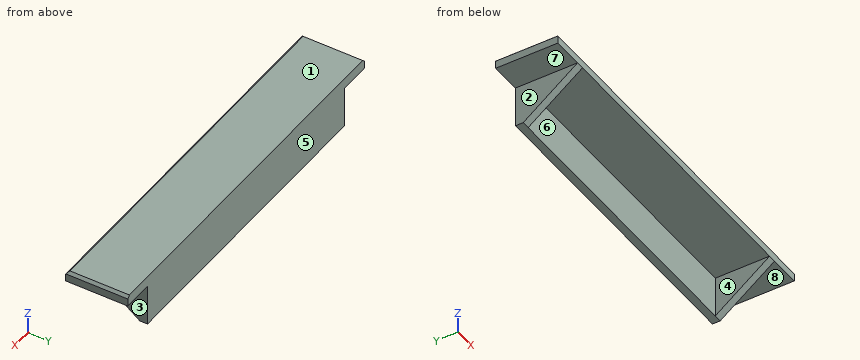
```python
from build123d import *

# Parameters (mm, degrees)
F0_W     = 914.4
F0_H     = 25.4
F1_DEPTH = 152.4
F2_SIZE  = 6.35
F3_W     = 19.05
F3_H     = 152.4
F4_DEPTH = 101.6
F6_DEPTH = 838.201
F7_W     = 19.05
F7_H     = 101.6
F8_DEPTH = 723.9


with BuildPart() as f1:
    # F0 (on Front) → F1 (new body)
    with BuildSketch(Plane.XZ):
        Rectangle(F0_W, F0_H)
    extrude(amount=F1_DEPTH)

    # F2
    f2_edges = [f1.edges().sort_by_distance(p)[0] for p in [
        (-457.2, -76.2, 12.7),
        (0, -152.4, 12.7),
        (457.2, -76.2, 12.7),
    ]]
    chamfer(f2_edges, length=F2_SIZE)

    # F3 (on face) → F4 (join)
    with BuildSketch(Plane(origin=(0, 0, -12.7), x_dir=(1, 0, 0), z_dir=(0, 0, -1))):
        with Locations((-371.475, 76.2)):
            Rectangle(F3_W, F3_H)
        with Locations((371.475, 76.2)):
            Rectangle(F3_W, F3_H)
    extrude(amount=F4_DEPTH)

    # F5 (on face) → F6 (cut, through all)
    with BuildSketch(Plane.YZ.offset(381)):
        Polygon((-19.05, -114.3), (-152.4, -12.7), (-152.4, -114.3), align=None)
    extrude(amount=-F6_DEPTH, mode=Mode.SUBTRACT)

    # F7 (on face) → F8 (join, through all)
    with BuildSketch(Plane.YZ.offset(-361.95)):
        with Locations((-9.525, -63.5)):
            Rectangle(F7_W, F7_H)
    extrude(amount=F8_DEPTH)


solid = f1.part
```
Read the model definition and answer for the solid it produces. Units are mm, in the model's axes. Face numbers are marked on the shaded views. A direction names the side the tool comes from. Give positions to 0.01 mm unless a question says otherwise; leave off trailing zeros. Loops run counter-clockwise (first coordinate to the right, second up) from the corner with the lowest first, then second, coordinate; pieces in that order, holes last.
Item 1: The part is cut by section A-A (z = -37.5). Write down the section's boundary in (x, y).
Item 2: Each of these flat-tipped pins is pushed along its axis until it touches: pin 1 Ø8 at (y, z) = (-15.5, -53.5) entering from -X; pin 2 Ø1.5 at (x, z) = (-191.5, -49.5) entering from -Y; pin 3 Ø3 at (x, y) = (305, -114.5) entering from -Z. Where does it stop, or does it pass through?
Item 3: The part is cut by section B-B (x = -189). Write down the section's boundary in (y, z), and give its area (3 significant figures).
Item 4: The part is cut by section D-D (x = 394). Write down the section's boundary in (y, z), and give its area (3 significant figures).
Item 5: Find the intervals of material crossed by line 1 along X through (y, z) = (-20, -34.5); line 2 along Z through (x, y) = (96.5, -59); line 3 along Y through (x, z) = (17, -22.5), in increasing order.
Item 6: The mould has two halves that part along X. Classify the marked faces 1, 2, 3 and 4: released by +X, released by -X, zero draft, split by the parting line, or undercut.
Item 7: For the marked faces 5, 6, 7 and 8, determine the directions among +Z, -Z, +X, -X, +Y, -Y from which every point of the face is accessible in a straight line to the end or side of a thin tool.
Item 8: The part is cut by section C-C (y = -114). Write down the section's boundary in (x, z).
Taken from the geometry:
1. outline: (-381, -119.85) - (-361.95, -119.85) - (-361.95, -19.05) - (361.95, -19.05) - (361.95, -119.85) - (381, -119.85) - (381, 0) - (-381, 0) - close
2. pin 1: stops at x = -381
2. pin 2: stops at y = -19.05
2. pin 3: stops at z = -12.7
3. outline: (-152.4, -12.7) - (-19.05, -12.7) - (-19.05, -114.3) - (0, -114.3) - (0, 12.7) - (-146.05, 12.7) - (-152.4, 6.35) - close
3. area: 5,790 mm2
4. outline: (-152.4, -12.7) - (0, -12.7) - (0, 12.7) - (-146.05, 12.7) - (-152.4, 6.35) - close
4. area: 3,850 mm2
5. line 1: x = -381 to -361.95, 361.95 to 381
5. line 2: z = -12.7 to 12.7
5. line 3: y = -19.05 to 0
6. face 1: zero draft
6. face 2: released by -X
6. face 3: released by +X
6. face 4: undercut
7. face 5: +Z, -Z, +X, -X, +Y
7. face 6: -Z, -Y
7. face 7: -Z, -X, +Y, -Y
7. face 8: -Z, +X, +Y, -Y
8. outline: (-457.2, -12.7) - (-381, -12.7) - (-381, -41.96) - (-361.95, -41.96) - (-361.95, -12.7) - (361.95, -12.7) - (361.95, -41.96) - (381, -41.96) - (381, -12.7) - (457.2, -12.7) - (457.2, 6.35) - (450.85, 12.7) - (-450.85, 12.7) - (-457.2, 6.35) - close
